```python
from build123d import *

# Parameters (mm, degrees)
F0_R      = 1.05
F1_DEPTH  = 1.3
F3_W      = 2.2
F3_H      = 23
F4_DEPTH  = 0.7
F5_W      = 2.5
F5_H      = 1.5
F5_W_2    = 3
F5_W_3    = 2.2
F5_H_2    = 23
F6_DEPTH  = 0.9
F7_R      = 0.3
F8_R      = 0.3
F9_W      = 2
F9_H      = 1
F9_H_2    = 14
F10_DEPTH = 0.9
F3_W_2    = 3
F3_H_2    = 1.5
F11_DEPTH = 0.9
F5_W_4    = 1.5
F5_H_3    = 2.5
F12_DEPTH = 1.8
F13_W     = 1.5
F13_H     = 2.5
F14_DEPTH = 0.5
F14_TAPER = -30
F3_W_3    = 1.5
F3_H_3    = 2.5
F15_DEPTH = 1.2
F16_W     = 1.5
F16_H     = 2.5
F17_DEPTH = 0.5
F17_TAPER = -30


with BuildPart() as f1:
    # F0 (on Top) → F1 (new body)
    with BuildSketch(Plane.XY):
        Polygon((21.3, -14), (32, -14), (32, 14), (21.3, 14), (21.3, 11.5), (19.1, 11.5), (19.1, 14), (1.3, 14), (1.3, 11.5), (-0.9, 11.5), (-0.9, 14), (-32, 14), (-32, -14), (-0.9, -14), (-0.9, -11.5), (1.3, -11.5), (1.3, -14), (19.1, -14), (19.1, -11.5), (21.3, -11.5), align=None)
        with Locations((-24.5, -11)):
            Circle(F0_R, mode=Mode.SUBTRACT)
        Polygon((-10, 7), (-10, 5.1), (-8.5, 5.1), (-8.5, 7), (11.5, 7), (11.5, 5.1), (29.6, 5.1), (29.6, -5.1), (11.5, -5.1), (11.5, -7), (-8.5, -7), (-8.5, -5.1), (-10, -5.1), (-10, -7), (-30.5, -7), (-30.5, -5.1), (-30.5, 5.1), (-30.5, 7), align=None, mode=Mode.SUBTRACT)
        with Locations((-24.5, 11)):
            Circle(F0_R, mode=Mode.SUBTRACT)
    extrude(amount=F1_DEPTH)

    # F3 (on face) → F4 (join)
    with BuildSketch(Plane.XY.offset(1.3)):
        with Locations((30.9, 0)):
            Rectangle(F3_W, F3_H)
    extrude(amount=F4_DEPTH)

    # F5 (on face) → F6 (join)
    with BuildSketch(Plane(origin=(0, 0, 0), x_dir=(1, 0, 0), z_dir=(0, 0, -1))):
        with Locations((-10.65, 12.3576217964)):
            Rectangle(F5_W, F5_H)
        with Locations((-10.65, -12.3576217964)):
            Rectangle(F5_W, F5_H)
        with Locations((24.5, -12.15)):
            Rectangle(F5_W_2, F5_H)
        with Locations((30.9, 0)):
            Rectangle(F5_W_3, F5_H_2)
        with Locations((24.5, 12.15)):
            Rectangle(F5_W_2, F5_H)
    extrude(amount=F6_DEPTH)

    # F7
    f7_edges = [f1.edges().sort_by_distance(p)[0] for p in [
        (32, 0, -0.9),
    ]]
    fillet(f7_edges, radius=F7_R)

    # F8
    f8_edges = [f1.edges().sort_by_distance(p)[0] for p in [
        (32, 0, 2),
    ]]
    fillet(f8_edges, radius=F8_R)

    # F9 (on face) → F10 (join)
    with BuildSketch(Plane(origin=(0, 0, 0), x_dir=(1, 0, 0), z_dir=(0, 0, -1))):
        with Locations((-20.5, 7.5)):
            Rectangle(F9_W, F9_H)
        with Locations((-20.5, -7.5)):
            Rectangle(F9_W, F9_H)
        with Locations((-20.5, 0)):
            Rectangle(F9_W, F9_H_2)
    extrude(amount=F10_DEPTH)

    # F3 (on face) → F11 (join)
    with BuildSketch(Plane.XY.offset(1.3)):
        with Locations((-10.4, 12.15)):
            Rectangle(F3_W_2, F3_H_2)
        with Locations((-10.4, -12.15)):
            Rectangle(F3_W_2, F3_H_2)
        with Locations((24.5, -12.15)):
            Rectangle(F3_W_2, F3_H_2)
        with Locations((24.5, 12.15)):
            Rectangle(F3_W_2, F3_H_2)
    extrude(amount=F11_DEPTH)

    # F5 (on face) → F12 (join)
    with BuildSketch(Plane(origin=(0, 0, 0), x_dir=(1, 0, 0), z_dir=(0, 0, -1))):
        with Locations((-14.15, 9.75)):
            Rectangle(F5_W_4, F5_H_3)
        with Locations((-14.15, -9.75)):
            Rectangle(F5_W_4, F5_H_3)
    extrude(amount=F12_DEPTH)

    # F13 (on face) → F14 (join)
    with BuildSketch(Plane(origin=(0, 0, -1.8), x_dir=(1, 0, 0), z_dir=(0, 0, -1))):
        with Locations((-14.15, 9.75)):
            Rectangle(F13_W, F13_H)
        with Locations((-14.15, -9.75)):
            Rectangle(F13_W, F13_H)
    extrude(amount=F14_DEPTH, taper=F14_TAPER)

    # F3 (on face) → F15 (join)
    with BuildSketch(Plane.XY.offset(1.3)):
        with Locations((-14.15, 9.75)):
            Rectangle(F3_W_3, F3_H_3)
        with Locations((-14.15, -9.75)):
            Rectangle(F3_W_3, F3_H_3)
    extrude(amount=F15_DEPTH)

    # F16 (on face) → F17 (join)
    with BuildSketch(Plane.XY.offset(2.5)):
        with Locations((-14.15, 9.75)):
            Rectangle(F16_W, F16_H)
        with Locations((-14.15, -9.75)):
            Rectangle(F16_W, F16_H)
    extrude(amount=F17_DEPTH, taper=F17_TAPER)


solid = f1.part
```
The listing builds one solid part. Answer for the finished solid, in the listing's coordinates (mm). A direction names the side the tool comes from. Coordinates: 2 decimals unless noted, no trailing zeros. Write each loop counter-clockwise with the first axis right and the second up, starting at its lowest first coordinate (ties: lowest second). Pieces come first, ordered by that corner, then holes.
Q1. Section C-C, the plane x = -5.5 is taken. Write down the section's boundary in (y, z), then the cut area to 3 significant figures.
Returned:
outline: (-14, 0) - (-7, 0) - (-7, 1.3) - (-14, 1.3) - close; (7, 0) - (14, 0) - (14, 1.3) - (7, 1.3) - close
area: 18.2 mm2
Q2. Given P1, Ø1.2, axis at x = -14, z = -1, coming from the +Y side; P2, Ø0.8, axis at x = 25, y = -12, coming from the +Z side; P3, Ø8, axis at x = 11.5, y = -10.5, coming from the -Z side; P4, Ø8, axis at x = 4.5, y = 2, coming from the +Z side, each flat-ended and moving along its own axis, determine where each tip first touches the part or whether it passes through.
Returned:
P1: stops at y = 11
P2: stops at z = 2.2
P3: stops at z = 0
P4: passes through
Q3. The mould has two halves that part along X. Classify faces 4 (the flat face through (31, 0, -0.9)), 5 (the flat face through (-0.9, -13, 1)), 6 (the flat face through (-13.4, 10, 2)), 7 (the flat face through (-14.9, -10, 2)): released by +X, released by -X, zero draft, split by the parting line, or undercut.
Returned:
face 4: zero draft
face 5: undercut
face 6: undercut
face 7: released by -X
Q4. Find the intervals of material crossed by line 1 along Y through (x, z) = (-24.5, 0.3); line 2 along X through (y, z) = (5.25, 0.35); line 3 along X through (y, z) = (10.5, -0.25), in increasing order.
Returned:
line 1: y = -14 to -12.05, -9.95 to -7, 7 to 9.95, 12.05 to 14
line 2: x = -32 to -30.5, -10 to -8.5, 11.5 to 32
line 3: x = -14.9 to -13.4, 29.8 to 32
Q5. Section A-A, the plane x = -24.5 is taken. Write down the section's boundary in (y, z), then the cut area to 3 significant figures.
Returned:
outline: (-14, 0) - (-12.05, 0) - (-12.05, 1.3) - (-14, 1.3) - close; (-9.95, 0) - (-7, 0) - (-7, 1.3) - (-9.95, 1.3) - close; (7, 0) - (9.95, 0) - (9.95, 1.3) - (7, 1.3) - close; (12.05, 0) - (14, 0) - (14, 1.3) - (12.05, 1.3) - close
area: 12.7 mm2
Q6. Section B-B, the plane y = -4.5 is taken. Write down the section's boundary in (x, z).
Returned:
outline: (-32, 0) - (-30.5, 0) - (-30.5, 1.3) - (-32, 1.3) - close; (-21.5, -0.9) - (-19.5, -0.9) - (-19.5, 0) - (-21.5, 0) - close; (29.6, 0) - (29.8, 0) - (29.8, -0.9) - (31.7, -0.9) arc R0.3 ccw to (32, -0.6) - (32, 1.7) arc R0.3 ccw to (31.7, 2) - (29.8, 2) - (29.8, 1.3) - (29.6, 1.3) - close
Q7. Which of the six approach directions +Z, -Z, +X, -X, +Y, -Y give full straight-line access (tool end or side, diameter ignored) to faces 1 (the flat face through (19.1, 13, 1)), 2 (the flat face through (-14, -11, 2)), 3 (the flat face through (-10, -6, 1))?
Returned:
face 1: +Z, -Z, +Y
face 2: -X, -Y
face 3: +Z, -Z
